from build123d import *

# Parameters (mm, degrees)
SKETCH2_W           = 220
SKETCH2_H           = 90
BOSS_EXTRUDE1_DEPTH = 4.5
SKETCH3_W           = 20.25
SKETCH3_H           = 6.5
CUT_EXTRUDE1_DEPTH  = 119.933805119
SKETCH5_R           = 1.65
BRACKET_HOLES_DEPTH = 119.933805119
SKETCH6_W           = 59.428711229
SKETCH6_H           = 112.188854202
TRIM_CUT_DEPTH      = 119.933805119


with BuildPart() as part:
    # Sketch2 → Boss-Extrude1 (new body)
    with BuildSketch(Plane(origin=(0, 0, 0), x_dir=(1, 0, 0), z_dir=(0, 1, 0))):
        Rectangle(SKETCH2_W, SKETCH2_H)
    extrude(amount=BOSS_EXTRUDE1_DEPTH)

    # Sketch3 → Cut-Extrude1 (cut, through all)
    with BuildSketch(Plane.XZ):
        with Locations((40, -15.925)):
            Rectangle(SKETCH3_W, SKETCH3_H)
        with Locations((0, -15.925)):
            Rectangle(SKETCH3_W, SKETCH3_H)
        with Locations((80, -15.925)):
            Rectangle(SKETCH3_W, SKETCH3_H)
        with Locations((-80, -15.925)):
            Rectangle(SKETCH3_W, SKETCH3_H)
        with Locations((-40, -15.925)):
            Rectangle(SKETCH3_W, SKETCH3_H)
        with Locations((-40, 35.925)):
            Rectangle(SKETCH3_W, SKETCH3_H)
        with Locations((-80, 35.925)):
            Rectangle(SKETCH3_W, SKETCH3_H)
        with Locations((80, 35.925)):
            Rectangle(SKETCH3_W, SKETCH3_H)
        with Locations((40, 35.925)):
            Rectangle(SKETCH3_W, SKETCH3_H)
        with Locations((0, 35.925)):
            Rectangle(SKETCH3_W, SKETCH3_H)
    extrude(amount=-CUT_EXTRUDE1_DEPTH, mode=Mode.SUBTRACT)

    # Sketch5 → Bracket holes (cut, through all)
    with BuildSketch(Plane.XZ):
        with Locations(Location((-26, 20.75, 0), (0, 0, 270))):
            Circle(SKETCH5_R)
        with Locations(Location((-14, 20.75, 0), (0, 0, 270))):
            Circle(SKETCH5_R)
        with Locations(Location((6.15, 20.75, 0), (0, 0, 270))):
            Circle(SKETCH5_R)
        with Locations(Location((54.65, 20.75, 0), (0, 0, 270))):
            Circle(SKETCH5_R)
        with Locations(Location((54.65, -0.75, 0), (0, 0, 90))):
            Circle(SKETCH5_R)
        with Locations(Location((6.15, -0.75, 0), (0, 0, 90))):
            Circle(SKETCH5_R)
        with Locations(Location((-14, -0.75, 0), (0, 0, 90))):
            Circle(SKETCH5_R)
        with Locations(Location((-26, -0.75, 0), (0, 0, 90))):
            Circle(SKETCH5_R)
    extrude(amount=-BRACKET_HOLES_DEPTH, mode=Mode.SUBTRACT)

    # Sketch6 → Trim cut (cut, through all)
    with BuildSketch(Plane.XZ):
        with Locations((-99.589355615, -2.07728242)):
            Rectangle(SKETCH6_W, SKETCH6_H)
    extrude(amount=-TRIM_CUT_DEPTH, mode=Mode.SUBTRACT)


solid = part.part
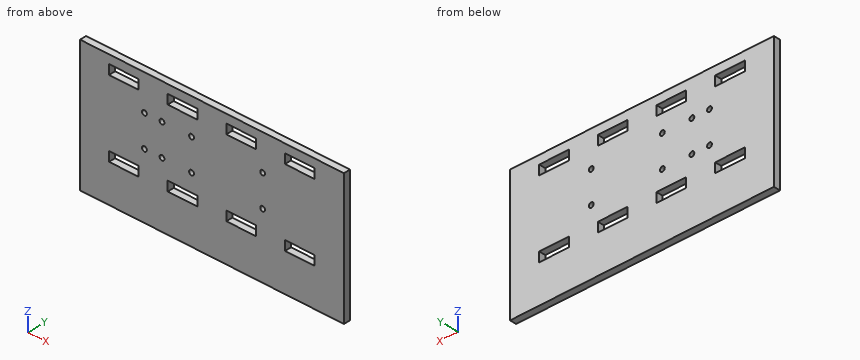
Read the model definition and answer for the solid it produces. Units are mm, in the model's axes. Round coordinates to 2 decimals unless told otherwise and drop trailing zeros. Write each loop counter-clockwise with the first axis right and the second up, starting at its lowest first coordinate (ties: lowest second). Pieces come first, ordered by that corner, then holes. Notation, with made-up numbers: M -33.5,8 L 20.5,8 A26 cw 20.5,35 Z; hole C 1.5,63 d3. An arc over 180 degrees is marked long. Use a Markdown table: item, result.
1) The part is cut by section B-B (x = -40). Write down the section's boundary in (y, z) (3 decimals).
Answers follow:
| item | result |
|---|---|
| outline | M 0,-45 L 4.5,-45 L 4.5,-19.175 L 0,-19.175 Z; M 0,-12.675 L 4.5,-12.675 L 4.5,32.675 L 0,32.675 Z; M 0,39.175 L 4.5,39.175 L 4.5,45 L 0,45 Z |
2) A flat-ended cylindrical pin translates along its axis: pin 1 (10 mm diameter, centred on x = -19.5, z = 0.5, fed in from -Y). Find the tip coordinate at first contact, or state that the pin passes through.
Answers follow:
| item | result |
|---|---|
| pin 1 | stops at y = 0 |
3) Straight lines are drawn through the part: line 1 along X through (y, z) = (2.35, 20.75) (3 decimals); line 2 along Z through (x, y) = (-48, 2.6) (3 decimals); line 3 along X through (y, z) = (2.9, 20) (3 decimals). For each, find the intervals that lie inside material, in ascending order. Write a range as [from, to].
Answers follow:
| item | result |
|---|---|
| line 1 | x = [-69.875, -27.65], [-24.35, -15.65], [-12.35, 4.5], [7.8, 53], [56.3, 110] |
| line 2 | z = [-45, -19.175], [-12.675, 32.675], [39.175, 45] |
| line 3 | x = [-69.875, -27.47], [-24.53, -15.47], [-12.53, 4.68], [7.62, 53.18], [56.12, 110] |
4) The part is cut by section C-C (x = 6.15). Write down the section's boundary in (y, z) (3 decimals).
Answers follow:
| item | result |
|---|---|
| outline | M 0,-45 L 4.5,-45 L 4.5,-19.175 L 0,-19.175 Z; M 0,-12.675 L 4.5,-12.675 L 4.5,-2.4 L 0,-2.4 Z; M 0,0.9 L 4.5,0.9 L 4.5,19.1 L 0,19.1 Z; M 0,22.4 L 4.5,22.4 L 4.5,32.675 L 0,32.675 Z; M 0,39.175 L 4.5,39.175 L 4.5,45 L 0,45 Z |
5) The part is cut by section D-D (x = -14). Write down the section's boundary in (y, z).
Answers follow:
| item | result |
|---|---|
| outline | M 0,-45 L 4.5,-45 L 4.5,-2.4 L 0,-2.4 Z; M 0,0.9 L 4.5,0.9 L 4.5,19.1 L 0,19.1 Z; M 0,22.4 L 4.5,22.4 L 4.5,45 L 0,45 Z |
6) The part is cut by section A-A (z = 20.75). Write down the section's boundary in (x, y) (3 decimals).
Answers follow:
| item | result |
|---|---|
| outline | M -69.875,0 L -27.65,0 L -27.65,4.5 L -69.875,4.5 Z; M -24.35,0 L -15.65,0 L -15.65,4.5 L -24.35,4.5 Z; M -12.35,0 L 4.5,0 L 4.5,4.5 L -12.35,4.5 Z; M 7.8,0 L 53,0 L 53,4.5 L 7.8,4.5 Z; M 56.3,0 L 110,0 L 110,4.5 L 56.3,4.5 Z |
